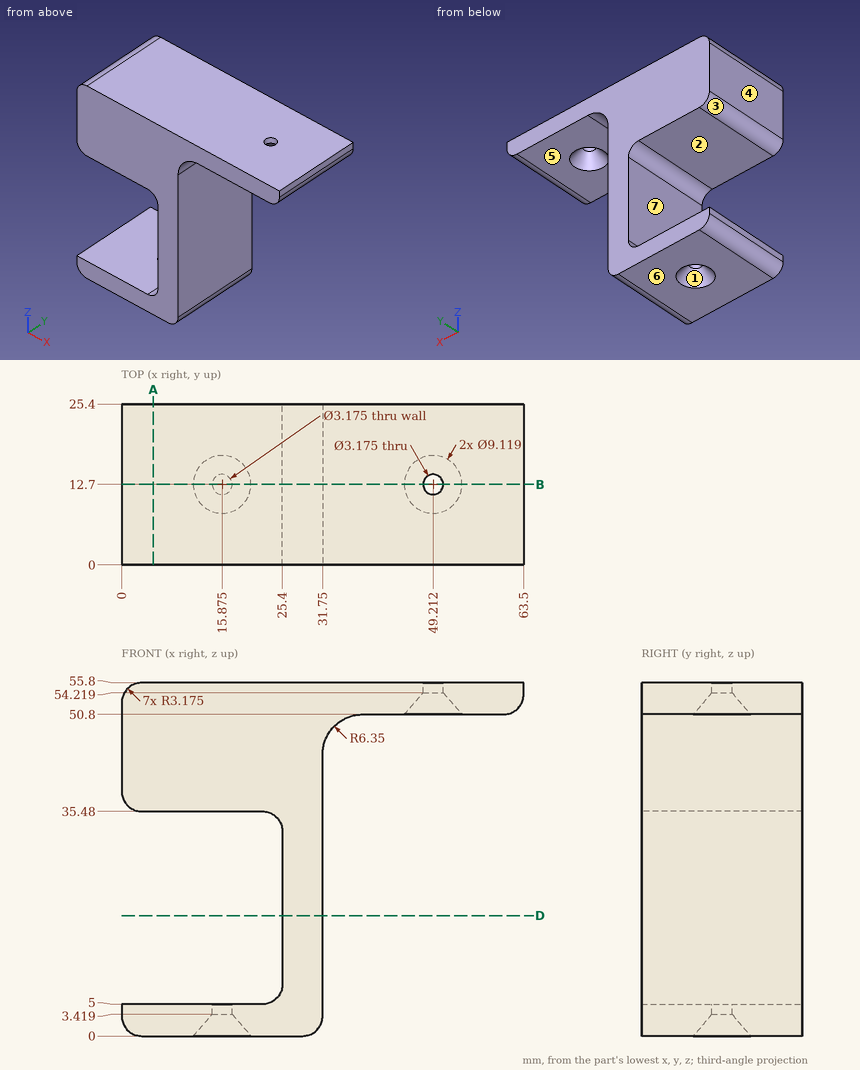
Verification items for this drawing (mm, ordinates from the low corner). A direction names the side the tool comes from. Coordinates: 2 decimals unless noted, no trailing zeros. Order: outer loops, then holes, each group sorted by start corner. A loop starts at its lowest first (then second) coordinate and runs counter-clockwise, first axis right, second up. Notation, with made-up numbers: (-23.5, -4) - (20.5, -4) arc R22 ccw to (20.5, 24) - close; hole circle Ø7 at (-8, 89.25). An arc over 180 degrees is marked (long way). Answer as a JSON object with one key per item and string values. Group by question number.
Item 1: Sectioned sample at B-B, the plane y = 12.7. Give the number of separate pieces and of enclosed holes in the cut face, and give its area (3 significant figures).
Item 2: Sectioned sample at A-A, the plane x = 5. Record the cut outline in (y, z), and give its area (3 significant figures).
Item 3: Depth check by flat-ended pin: pin 1 Ø12 at (x, y) = (38.5, 3.5) entering from -Z (1 decimal); pin 2 Ø4 at (x, y) = (15.875, 12.7) entering from -Z (1 decimal); pin 3 Ø1 at (y, z) = (8.5, 38.5) entering from +X. Enter the tip coordinate at first touch or a pass-through.
Item 4: Tool access check on the marked faces 5, 6 and 7. Record the directions out of +Z, -Z, +X, -X, +Y, -Y that give a thin tool (end or side, any length) a straight path to the whole face; none if there is none.
Item 5: Draft check along Z on the marked faces 1, 2, 3 and 4. Enter one of: +Z half, -Z half, draft (parallel to the pull), parting line (faces both ways), or undercut.
Item 6: Scan lines: probe 1 along X at (y, z) = (12.7, 3.95); probe 2 along Z at (x, y) = (57.5, 19); probe 3 along Z at (x, y) = (15.5, 22.5). Record each from-to range of solid material in increasing order.
Item 7: Sectioned sample at D-D, the plane z = 19. Record the cut outline in (x, y).
Resolved:
{
 "1": {"separate pieces": "3", "enclosed holes": "0", "area": "1,110 mm^2"},
 "2": {"outline": "(0, 0) - (25.4, 0) - (25.4, 5) - (0, 5) - close; (0, 35.48) - (25.4, 35.48) - (25.4, 55.8) - (0, 55.8) - close", "area": "643 mm^2"},
 "3": {"pin 1": "z = 47.4", "pin 2": "z = 2.9", "pin 3": "x = 31.75"},
 "4": {"face 5": "-Z, +X, +Y, -Y", "face 6": "-Z, +X, -X, +Y, -Y", "face 7": "-X, +Y, -Y"},
 "5": {"face 1": "-Z half", "face 2": "undercut", "face 3": "undercut", "face 4": "draft"},
 "6": {"probe 1": "0 to 14.29, 17.46 to 31.75", "probe 2": "50.8 to 55.8", "probe 3": "0 to 5, 35.48 to 55.8"},
 "7": {"outline": "(25.4, 0) - (31.75, 0) - (31.75, 25.4) - (25.4, 25.4) - close"}
}
